from build123d import *

# Parameters (mm, degrees)
F0_W     = 30
F0_H     = 15
F1_DEPTH = 3
F2_W     = 30
F2_H     = 2.5
F3_DEPTH = 5
F4_R     = 3


with BuildPart() as f1:
    # F0 (on Top) → F1 (new body)
    with BuildSketch(Plane.XY):
        Rectangle(F0_W, F0_H)
    extrude(amount=F1_DEPTH)

    # F2 (on face) → F3 (join)
    with BuildSketch(Plane.XY.offset(3)):
        with Locations((0, 6.25)):
            Rectangle(F2_W, F2_H)
        with Locations((0, -6.25)):
            Rectangle(F2_W, F2_H)
    extrude(amount=F3_DEPTH)

    # F4
    f4_edges = [f1.edges().sort_by_distance(p)[0] for p in [
        (0, 5, 3),
        (0, -5, 3),
        (0, 7.5, 0),
        (0, -7.5, 0),
    ]]
    fillet(f4_edges, radius=F4_R)


solid = f1.part
Part model, mm, in its own coordinate system. A direction names the side the tool comes from. Coordinates: 2 decimals unless noted, no trailing zeros. Order: outer loops, then holes, each group sorted by start corner. A loop starts at its lowest first (then second) coordinate and runs counter-clockwise, first axis right, second up. Notation, with made-up numbers: M 38,14.25 L 60,14.25 A7 ccw 60,22.25 Z; hole C -29,89.25 d8. An arc over 180 degrees is marked long. Use a Markdown table: item, result.
(1) Flat gauge pin, fed straight in: pin 1 (3 mm diameter, centred on x = 6.5, y = 1, fed in from +Z). Where does the tip first touch, or does it go through?
A:
| item | result |
|---|---|
| pin 1 | stops at z = 3.04 |
(2) Cut at B-B on x = 11.5. Write the cut outline in (y, z).
A:
| item | result |
|---|---|
| outline | M -7.5,3 A3 ccw -4.5,0 L 4.5,0 A3 ccw 7.5,3 L 7.5,8 L 5,8 L 5,6 A3 cw 2,3 L -2,3 A3 cw -5,6 L -5,8 L -7.5,8 Z |
(3) Tool access for faces 4 (the flat face through (15, 0, 2)), 5 (the flat face through (0, 0, 3)): list every direction of +Z, -Z, +X, -X, +Y, -Y with a clear straight run to the whole face (end or side of a thin tool).
A:
| item | result |
|---|---|
| face 4 | +Z, -Z, +X, +Y, -Y |
| face 5 | +Z, +X, -X |
(4) Cut at D-D on y = 1.5. Write the cut outline in (x, z), then the cut area to 3 significant figures.
A:
| item | result |
|---|---|
| outline | M -15,0 L 15,0 L 15,3 L -15,3 Z |
| area | 90.0 mm^2 |
(5) Probe L1, parallel to Y at x = 9, z = 7; L2, parallel to Z at x = 7.25, y = 0; L3, parallel to Y at x = -13.5, z = 5. List the from-to ranges inside material, lowest first.
A:
| item | result |
|---|---|
| L1 | y = -7.5 to -5, 5 to 7.5 |
| L2 | z = 0 to 3 |
| L3 | y = -7.5 to -4.83, 4.83 to 7.5 |
(6) Cut at A-A on z = 7. Write the cut outline in (x, y), then the cut area to 3 significant figures.
A:
| item | result |
|---|---|
| outline | M -15,-7.5 L 15,-7.5 L 15,-5 L -15,-5 Z; M -15,5 L 15,5 L 15,7.5 L -15,7.5 Z |
| area | 150 mm^2 |
(7) Cut at C-C on z = 5.25. Write the cut outline in (x, y).
A:
| item | result |
|---|---|
| outline | M -15,-7.5 L 15,-7.5 L 15,-4.9 L -15,-4.9 Z; M -15,4.9 L 15,4.9 L 15,7.5 L -15,7.5 Z |
(8) Pull direction Y, two halves, no side cores. Call faces 1 (the cylindrical face through (0.21, 6.6, 0.86)), 2 (the cylindrical face through (0.21, 4.1, 3.86)), 3 (the flat face through (0, 0, 0)): released by +Y, released by -Y, zero draft, split by the parting line, or undercut.
A:
| item | result |
|---|---|
| face 1 | released by +Y |
| face 2 | undercut |
| face 3 | zero draft |
